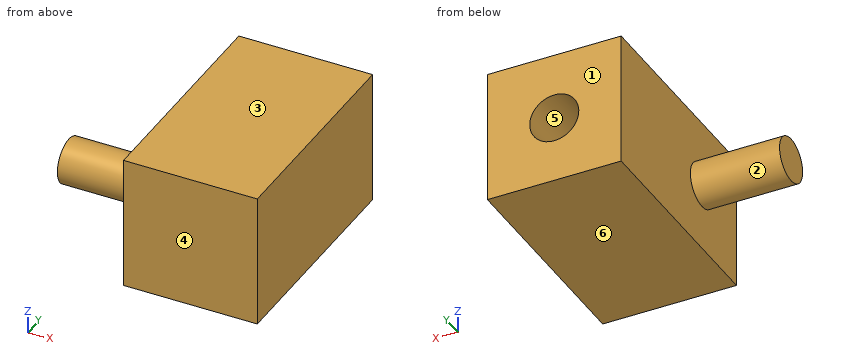
from build123d import *

# Parameters (mm, degrees)
SKETCH1_W           = 76.2
SKETCH1_H           = 127
BOSS_EXTRUDE1_DEPTH = 76.2
SKETCH2_R           = 13.97
CUT_EXTRUDE1_DEPTH  = 48.26
SKETCH3_R           = 12.7
BOSS_EXTRUDE2_DEPTH = 50.8


with BuildPart() as part:
    # Sketch1 → Boss-Extrude1 (new body)
    with BuildSketch(Plane.XY):
        Rectangle(SKETCH1_W, SKETCH1_H)
    extrude(amount=BOSS_EXTRUDE1_DEPTH)

    # Sketch2 → Cut-Extrude1 (cut)
    with BuildSketch(Plane(origin=(0, 63.5, 0), x_dir=(1, 0, 0), z_dir=(0, 1, 0))):
        with Locations(Location((0, -38.1, 0), (0, 0, 270))):
            Circle(SKETCH2_R)
    extrude(amount=-CUT_EXTRUDE1_DEPTH, mode=Mode.SUBTRACT)

    # Sketch3 → Boss-Extrude2 (add)
    with BuildSketch(Plane.ZY.offset(38.1)):
        with Locations(Location((38.1, -25.4, 0), (0, 0, 270))):
            Circle(SKETCH3_R)
    extrude(amount=BOSS_EXTRUDE2_DEPTH)


solid = part.part
Build history of the part. All positions in model axes, mm. Face numbers are marked on the shaded views. A direction names the side the tool comes from. Round coordinates to 2 decimals unless told otherwise and drop trailing zeros. Loops run counter-clockwise (first coordinate to the right, second up) from the corner with the lowest first, then second, coordinate; pieces in that order, holes last. Notation, with made-up numbers: (-38.5, 19) -> (5.5, 19) arc R20 ccw to (5.5, 43) -> close; hole circle Ø7 at (0.25, -36.75). An arc over 180 degrees is marked (long way). One line per item, written item: value. Start each with the question number.
Q1. Two-plate mould, pull along Y, no slides. Class the marked faces 1, 2, 3 and 4: released by +Y, released by -Y, zero draft, split by the parting line, or undercut.
Q2. Cut at A-A on y = 18. List the corners of the cut face in (x, z), plus the area to 3 significant figures.
Q3. Cut at D-D on z = 38.1. List the corners of the cut face in (x, y), plus the area to 3 significant figures.
Q4. Drop flat-ended pins along their axis: pin 1 Ø2 at (x, y) = (23.5, -23) entering from -Z; pin 2 Ø3 at (y, z) = (25, 34) entering from -X; pin 3 Ø6 at (x, y) = (-46.5, -32) entering from -Z. Give the stop position or say it passes through.
Q5. 3-axis set-ups, long thin cutter, end or side, ignore diameter. For the marked faces 5 and 6: which of +Z, -Z, +X, -X, +Y, -Y reach the whole face in a straight line?
Q6. Probe line 1 along X through (y, z) = (31, 38.1); line 2 along X through (y, z) = (37, 68); line 3 along Y through (x, z) = (2, 25.5). List the from-to ranges inside material, lowest first.
Q7. Cut at C-C on y = -25.4. List the corners of the cut face in (x, z), plus the area to 3 significant figures.
Computed:
1. face 1: released by +Y
1. face 2: split by the parting line
1. face 3: zero draft
1. face 4: released by -Y
2. outline: (-38.1, 0) -> (38.1, 0) -> (38.1, 76.2) -> (-38.1, 76.2) -> close; hole circle Ø27.94 at (0, 38.1)
2. area: 5,190 mm²
3. outline: (-88.9, -38.1) -> (-38.1, -38.1) -> (-38.1, -63.5) -> (38.1, -63.5) -> (38.1, 63.5) -> (13.97, 63.5) -> (13.97, 15.24) -> (-13.97, 15.24) -> (-13.97, 63.5) -> (-38.1, 63.5) -> (-38.1, -12.7) -> (-88.9, -12.7) -> close
3. area: 9,620 mm²
4. pin 1: z = 0
4. pin 2: x = -38.1
4. pin 3: z = 25.92
5. face 5: +Y
5. face 6: -Z, +X, -X, +Y, -Y
6. line 1: -38.1 to -13.97, 13.97 to 38.1
6. line 2: -38.1 to 38.1
6. line 3: -63.5 to 15.24
7. outline: (-88.9, 25.4) -> (-38.1, 25.4) -> (-38.1, 0) -> (38.1, 0) -> (38.1, 76.2) -> (-38.1, 76.2) -> (-38.1, 50.8) -> (-88.9, 50.8) -> close
7. area: 7,100 mm²
